Here's the drawing with two shaded views (mm, measured from the low corner). I have some questions. Coordinates: 2 decimals unless noted, no trailing zeros. Loops run counter-clockwise (first coordinate to the right, second up) from the corner with the lowest first, then second, coordinate; pieces in that order, holes last.
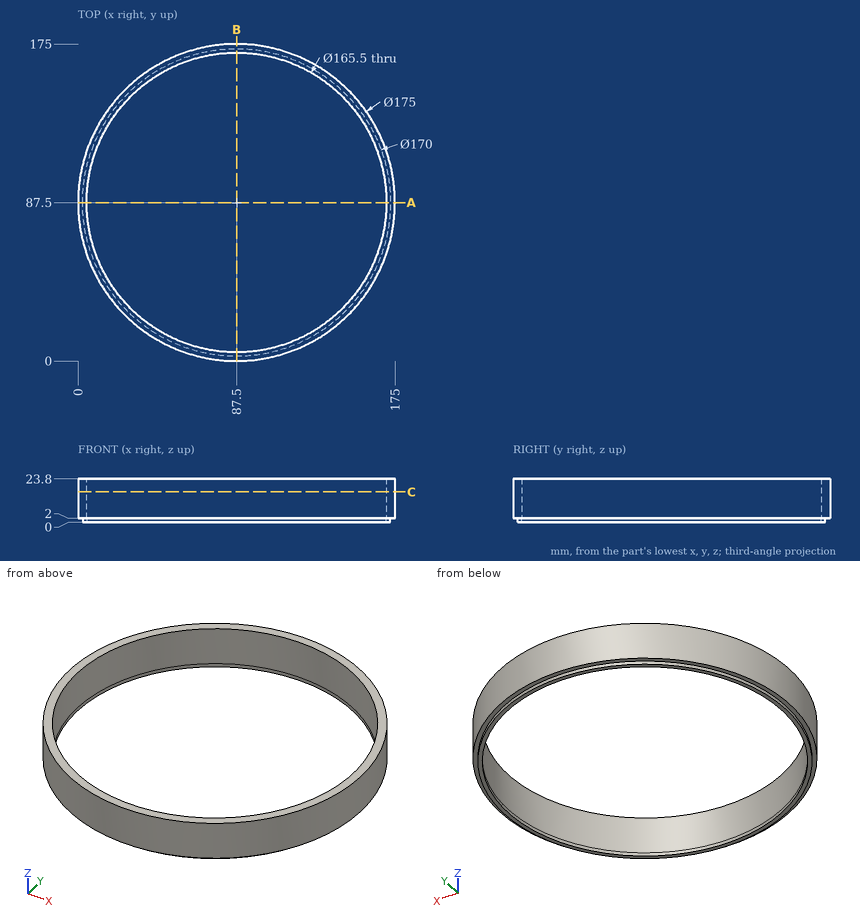
Q1. Suppose I cut it at C-C on z = 16.75. Write out the boundary of the cut face in (x, y), and give its area (3 significant figures).
Q2. Suppose I cut it at A-A on y = 87.5. Write out the boundary of the cut face in (x, z).
Q3. Please list where these lines run through material, in increasing order: probe 1 along Y at (x, z) = (87.5, 9); probe 2 along Y at (x, z) = (87.5, 0.7); probe 3 along X at (y, z) = (36.5, 5).
Q4. Will these pins go through, and if not, where does the flat tip stop? P1, Ø10, axis at x = 137.5, z = 5.5, coming from the +Y side; P2, Ø8, axis at y = 34.5, z = 12, coming from the +X side; P3, Ø1, axis at y = 21, z = 4.5, coming from the +X side.
Check values:
1. outline: circle Ø175 at (87.5, 87.5); hole circle Ø165.5 at (87.5, 87.5)
1. area: 2,540 mm2
2. outline: (0, 2) - (2.5, 2) - (2.5, 0) - (4.75, 0) - (4.75, 23.8) - (0, 23.8) - close; (170.25, 0) - (172.5, 0) - (172.5, 2) - (175, 2) - (175, 23.8) - (170.25, 23.8) - close
3. probe 1: y = 0 to 4.75, 170.25 to 175
3. probe 2: y = 2.5 to 4.75, 170.25 to 172.5
3. probe 3: x = 16.4 to 22.33, 152.67 to 158.6
4. P1: stops at y = 162.54
4. P2: stops at x = 159.99
4. P3: stops at x = 144.95
